Source: CAD feature listing. Evaluate the final solid. Frame: model axes, mm. Face numbers are marked on the shaded views. A direction names the side the tool comes from. Coordinates: 2 decimals unless noted, no trailing zeros. Write each loop counter-clockwise with the first axis right and the second up, starting at its lowest first coordinate (ties: lowest second). Pieces come first, ordered by that corner, then holes. Notation, with made-up numbers: (63.5, 63) -> (73.5, 63) arc R26 ccw to (73.5, 98) -> close; hole circle Ø8 at (-1, 44). An arc over 180 degrees is marked (long way). Write item = value, one per line.
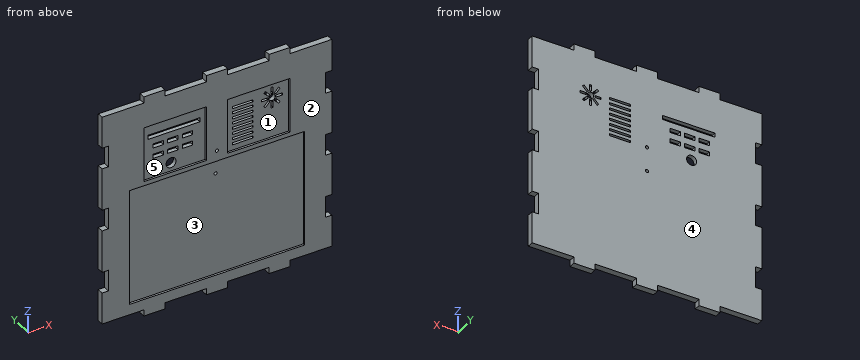
from build123d import *

# Parameters (mm, degrees)
F0_W     = 10
F0_H     = 3
F1_DEPTH = 3
F2_R     = 0.75
F2_W     = 5
F2_H     = 2
F2_R_2   = 2.4
F2_W_2   = 25
F2_W_3   = 10
F2_H_2   = 1
F2_R_3   = 1.5
F3_DEPTH = 3
F2_W_4   = 30
F2_H_3   = 26
F4_DEPTH = 1


# Not quite as in the source:
# - a feature names something its author has since deleted; it is built from what else it names


with BuildPart() as f1:
    # F0 (on Front) → F1 (new body)
    with BuildSketch(Plane.XZ):
        with Locations((-30, 51.5)):
            Rectangle(F0_W, F0_H)
        with Locations((0, 51.5)):
            Rectangle(F0_W, F0_H)
        with Locations((30, 51.5)):
            Rectangle(F0_W, F0_H)
        with Locations((-30, 48.5)):
            Rectangle(F0_W, F0_H)
        with Locations((0, 48.5)):
            Rectangle(F0_W, F0_H)
        with Locations((30, 48.5)):
            Rectangle(F0_W, F0_H)
        Polygon((-35, 50), (-55, 50), (-55, 35), (-52, 35), (-52, 25), (-55, 25), (-55, 5), (-52, 5), (-52, -5), (-55, -5), (-55, -25), (-52, -25), (-52, -35), (-55, -35), (-55, -50), (-35, -50), (-35, -47), (-25, -47), (-25, -50), (-5, -50), (-5, -47), (5, -47), (5, -50), (25, -50), (25, -47), (35, -47), (35, -50), (55, -50), (55, -35), (52, -35), (52, -25), (55, -25), (55, -5), (52, -5), (52, 5), (55, 5), (55, 25), (52, 25), (52, 35), (55, 35), (55, 50), (35, 50), (35, 47), (25, 47), (25, 50), (5, 50), (5, 47), (-5, 47), (-5, 50), (-25, 50), (-25, 47), (-35, 47), align=None)
        with Locations((30, -48.5)):
            Rectangle(F0_W, F0_H)
        with Locations((30, -51.5)):
            Rectangle(F0_W, F0_H)
        with Locations((0, -48.5)):
            Rectangle(F0_W, F0_H)
        with Locations((0, -51.5)):
            Rectangle(F0_W, F0_H)
        with Locations((-30, -48.5)):
            Rectangle(F0_W, F0_H)
        with Locations((-30, -51.5)):
            Rectangle(F0_W, F0_H)
    extrude(amount=F1_DEPTH)

    # F2 (on face) → F3 (cut)
    with BuildSketch(Plane.XZ.offset(3)):
        with Locations((0, 15)):
            Circle(F2_R)
        with Locations((-13.5, 22)):
            Rectangle(F2_W, F2_H)
        with Locations((-20.5, 22)):
            Rectangle(F2_W, F2_H)
        with Locations((-21.369388327, 16)):
            Circle(F2_R_2)
        with Locations((-27.5, 22)):
            Rectangle(F2_W, F2_H)
        with Locations((-27.5, 27)):
            Rectangle(F2_W, F2_H)
        with Locations((-20.5, 27)):
            Rectangle(F2_W, F2_H)
        with Locations((-13.5, 27)):
            Rectangle(F2_W, F2_H)
        with Locations((-20, 32)):
            Rectangle(F2_W_2, F2_H)
        with Locations((13, 32.5)):
            Rectangle(F2_W_3, F2_H_2)
        with Locations((13, 30)):
            Rectangle(F2_W_3, F2_H_2)
        with Locations((13, 27.5)):
            Rectangle(F2_W_3, F2_H_2)
        with Locations((13, 25)):
            Rectangle(F2_W_3, F2_H_2)
        with Locations((13, 22.5)):
            Rectangle(F2_W_3, F2_H_2)
        with Locations((13, 20)):
            Rectangle(F2_W_3, F2_H_2)
        with Locations((13, 17.5)):
            Rectangle(F2_W_3, F2_H_2)
        with Locations((13, 15)):
            Rectangle(F2_W_3, F2_H_2)
        with Locations((0, 3.5)):
            Circle(F2_R)
        Polygon((28.0606601718, 32.767766953), (28.4142135865, 32.4142135383), (28.767766953, 32.0606601718), (30.8890872965, 34.1819805153), (30.1819805153, 34.8890872965), align=None)
        Polygon((26.5, 33), (27, 33), (27.5, 33), (27.5, 36), (26.5, 36), align=None)
        Polygon((25.232233047, 32.0606601718), (25.5857864376, 32.4142135624), (25.9393398282, 32.767766953), (23.8180194847, 34.8890872965), (23.1109127035, 34.1819805153), align=None)
        Polygon((25, 30.5), (25, 31), (25, 31.5), (22, 31.5), (22, 30.5), align=None)
        Polygon((25.9393398282, 29.232233047), (25.5857864376, 29.5857864376), (25.232233047, 29.9393398282), (23.1109127035, 27.8180194847), (23.8180194847, 27.1109127035), align=None)
        Polygon((27.5, 29), (27, 29), (26.5, 29), (26.5, 26), (27.5, 26), align=None)
        Polygon((28.767766953, 29.9393398282), (28.4142135624, 29.5857864376), (28.0606601718, 29.232233047), (30.1819805153, 27.1109127035), (30.8890872965, 27.8180194847), align=None)
        Polygon((29, 31.5), (29, 31), (29, 30.5), (32, 30.5), (32, 31.5), align=None)
        with Locations((27, 31)):
            Circle(F2_R_3)
    extrude(amount=-F3_DEPTH, mode=Mode.SUBTRACT)

    # F2 (on face) → F4 (cut)
    with BuildSketch(Plane.XZ.offset(3)):
        with Locations((20, 25)):
            Rectangle(F2_W_4, F2_H_3)
        with Locations((13, 15)):
            Rectangle(F2_W_3, F2_H_2, mode=Mode.SUBTRACT)
        with Locations((13, 17.5)):
            Rectangle(F2_W_3, F2_H_2, mode=Mode.SUBTRACT)
        with Locations((13, 20)):
            Rectangle(F2_W_3, F2_H_2, mode=Mode.SUBTRACT)
        with Locations((13, 22.5)):
            Rectangle(F2_W_3, F2_H_2, mode=Mode.SUBTRACT)
        with Locations((13, 25)):
            Rectangle(F2_W_3, F2_H_2, mode=Mode.SUBTRACT)
        with Locations((13, 27.5)):
            Rectangle(F2_W_3, F2_H_2, mode=Mode.SUBTRACT)
        with Locations((13, 30)):
            Rectangle(F2_W_3, F2_H_2, mode=Mode.SUBTRACT)
        with Locations((13, 32.5)):
            Rectangle(F2_W_3, F2_H_2, mode=Mode.SUBTRACT)
        Polygon((26.5, 29), (27, 29), (27.5, 29), (27.5, 26), (26.5, 26), align=None, mode=Mode.SUBTRACT)
        Polygon((25.232233047, 29.9393398282), (25.5857864376, 29.5857864376), (25.9393398282, 29.232233047), (23.8180194847, 27.1109127035), (23.1109127035, 27.8180194847), align=None, mode=Mode.SUBTRACT)
        Polygon((25, 31.5), (25, 31), (25, 30.5), (22, 30.5), (22, 31.5), align=None, mode=Mode.SUBTRACT)
        with BuildLine():
            ThreePointArc((28.4142135865, 32.4142135383), (28.8477590715, 31.765366849), (29, 31))
            ThreePointArc((29, 31), (28.847759065, 30.2346331353), (28.4142135624, 29.5857864376))
            ThreePointArc((28.4142135624, 29.5857864376), (27.7653668647, 29.152240935), (27, 29))
            ThreePointArc((27, 29), (26.2346331353, 29.152240935), (25.5857864376, 29.5857864376))
            ThreePointArc((25.5857864376, 29.5857864376), (25.152240935, 30.2346331353), (25, 31))
            ThreePointArc((25, 31), (25.152240935, 31.7653668647), (25.5857864376, 32.4142135624))
            ThreePointArc((25.5857864376, 32.4142135624), (26.2346331353, 32.847759065), (27, 33))
            ThreePointArc((27, 33), (27.7653668805, 32.8477590585), (28.4142135865, 32.4142135383))
        make_face(mode=Mode.SUBTRACT)
        Polygon((25.9393398282, 32.767766953), (25.5857864376, 32.4142135624), (25.232233047, 32.0606601718), (23.1109127035, 34.1819805153), (23.8180194847, 34.8890872965), align=None, mode=Mode.SUBTRACT)
        Polygon((27.5, 33), (27, 33), (26.5, 33), (26.5, 36), (27.5, 36), align=None, mode=Mode.SUBTRACT)
        Polygon((28.0606601718, 29.232233047), (28.4142135624, 29.5857864376), (28.767766953, 29.9393398282), (30.8890872965, 27.8180194847), (30.1819805153, 27.1109127035), align=None, mode=Mode.SUBTRACT)
        Polygon((29, 30.5), (29, 31), (29, 31.5), (32, 31.5), (32, 30.5), align=None, mode=Mode.SUBTRACT)
        Polygon((28.767766953, 32.0606601718), (28.4142135865, 32.4142135383), (28.0606601718, 32.767766953), (30.1819805153, 34.8890872965), (30.8890872965, 34.1819805153), align=None, mode=Mode.SUBTRACT)
        with Locations((-20, 25)):
            Rectangle(F2_W_4, F2_H_3)
        with Locations((-21.369388327, 16)):
            Circle(F2_R_2, mode=Mode.SUBTRACT)
        with Locations((-27.5, 22)):
            Rectangle(F2_W, F2_H, mode=Mode.SUBTRACT)
        with Locations((-20.5, 22)):
            Rectangle(F2_W, F2_H, mode=Mode.SUBTRACT)
        with Locations((-13.5, 22)):
            Rectangle(F2_W, F2_H, mode=Mode.SUBTRACT)
        with Locations((-27.5, 27)):
            Rectangle(F2_W, F2_H, mode=Mode.SUBTRACT)
        with Locations((-20.5, 27)):
            Rectangle(F2_W, F2_H, mode=Mode.SUBTRACT)
        with Locations((-20, 32)):
            Rectangle(F2_W_2, F2_H, mode=Mode.SUBTRACT)
        with Locations((-13.5, 27)):
            Rectangle(F2_W, F2_H, mode=Mode.SUBTRACT)
        with BuildLine():
            ThreePointArc((28.4142135624, 29.5857864376), (28.847759065, 30.2346331353), (29, 31))
            ThreePointArc((29, 31), (28.8477590715, 31.765366849), (28.4142135865, 32.4142135383))
            ThreePointArc((28.4142135865, 32.4142135383), (27.7653668805, 32.8477590585), (27, 33))
            ThreePointArc((27, 33), (26.2346331353, 32.847759065), (25.5857864376, 32.4142135624))
            ThreePointArc((25.5857864376, 32.4142135624), (25.152240935, 31.7653668647), (25, 31))
            ThreePointArc((25, 31), (25.152240935, 30.2346331353), (25.5857864376, 29.5857864376))
            ThreePointArc((25.5857864376, 29.5857864376), (26.2346331353, 29.152240935), (27, 29))
            ThreePointArc((27, 29), (27.7653668647, 29.152240935), (28.4142135624, 29.5857864376))
        make_face()
        with Locations((27, 31)):
            Circle(F2_R_3, mode=Mode.SUBTRACT)
        Polygon((-35, 10), (-42, 10), (-42, -45), (42, -45), (42, 10), (35, 10), (5, 10), (-5, 10), align=None)
        with Locations((0, 3.5)):
            Circle(F2_R, mode=Mode.SUBTRACT)
    extrude(amount=-F4_DEPTH, mode=Mode.SUBTRACT)


solid = f1.part
1) First-contact query: pin 1 Ø1.5 at (y, z) = (-2, 51.5) entering from -X; pin 2 Ø1 at (x, y) = (14.5, -1) entering from +Z; pin 3 Ø1.6 at (x, y) = (13.5, -0.5) entering from -Z. Flat tips, straight axial feed; report the tip coordinate or a pass-through.
Answer block:
pin_1 = -35
pin_2 = 50
pin_3 = -50
2) Cut plane C-C, the plane x = 44. Output: boundary loops of the cut face in (y, z), and give its area (3 significant figures).
Answer block:
outline = (-3, -50) -> (0, -50) -> (0, 50) -> (-3, 50) -> close
area = 300 mm2
3) Pull-direction query (X, two-part tool) for the marked faces 3, 4 and 5; classes: +X half, -X half, draft (parallel to the pull), parting line (faces both ways), or undercut.
Answer block:
face_3 = undercut
face_4 = draft
face_5 = undercut
4) Reachability of the marked faces 1 and 2 from +Z, -Z, +X, -X, +Y, -Y: full face, straight path, thin tool, end or side. Return the list, or none.
Answer block:
face_1 = -Y
face_2 = +Z, -Z, +X, -X, -Y
5) Cut plane A-A, the plane z = -36.5. Output: boundary loops of the cut face in (x, y).
Answer block:
outline = (-55, -3) -> (-42, -3) -> (-42, -2) -> (42, -2) -> (42, -3) -> (55, -3) -> (55, 0) -> (-55, 0) -> close
6) Cut plane B-B, the plane y = -0.65. Give the number of separate pieces and of enclosed holes in the cut face, and give its area (3 significant figures).
Answer block:
separate_pieces = 1
enclosed_holes = 27
area = 10,800 mm2
7) Cut plane D-D, the plane z = -1. Output: boundary loops of the cut face in (x, y).
Answer block:
outline = (-52, -3) -> (-42, -3) -> (-42, -2) -> (42, -2) -> (42, -3) -> (52, -3) -> (52, 0) -> (-52, 0) -> close
8) Material intervals for probe 1 along Z at (x, y) = (-13.5, -0.85); probe 2 along Z at (x, y) = (16, -2.5); probe 3 along Z at (x, y) = (27, -1), sorted ascending. Write a range as [from, to].
Answer block:
probe_1 = [-50, 21], [23, 26], [28, 31], [33, 50]
probe_2 = [-50, -45], [10, 12], [38, 50]
probe_3 = [-53, 26], [29, 29.5], [32.5, 33], [36, 53]
